from build123d import *

# Parameters (mm, degrees)
F1_DEPTH = 10
F3_DEPTH = 15
F4_R     = 0.99999


# Not quite as in the source:
# - a fillet or chamfer is up to 0.001 mm smaller than in the source, because OpenCascade refuses the exact size


with BuildPart() as f1:
    # F0 (on Top) → F1 (new body)
    with BuildSketch(Plane.XY):
        with BuildLine():
            ThreePointArc((-6.7175144213, -6.7175144213), (0, 9.5), (6.7175144213, -6.7175144213))
            Line((6.7175144213, -6.7175144213), (8.1317279836, -8.1317279836))
            ThreePointArc((8.1317279836, -8.1317279836), (11.4919258811, 0.430859077), (7.5, 8.7177978871))
            Line((7.5, 8.7177978871), (7.5, 9.5))
            Line((7.5, 9.5), (7.5, 14.5))
            Line((7.5, 14.5), (-7.5, 14.5))
            Line((-7.5, 14.5), (-7.5, 9.5))
            Line((-7.5, 9.5), (-7.5, 8.7177978871))
            ThreePointArc((-7.5, 8.7177978871), (-11.4919258811, 0.430859077), (-8.1317279836, -8.1317279836))
            Line((-8.1317279836, -8.1317279836), (-6.7175144213, -6.7175144213))
        make_face()
    extrude(amount=F1_DEPTH)

    # F2 (on face) → F3 (join, through all)
    with BuildSketch(Plane.YZ.offset(7.5)):
        with BuildLine():
            ThreePointArc((14.5, 5), (15.0465956117, 7.7117470016), (16.6010205144, 10))
            Line((16.6010205144, 10), (14.5, 10))
            Line((14.5, 10), (14.5, 5))
        make_face()
        with BuildLine():
            Line((14.5, 0), (16.6010205144, 0))
            ThreePointArc((16.6010205144, 0), (15.0465956117, 2.2882529984), (14.5, 5))
            Line((14.5, 5), (14.5, 0))
        make_face()
    extrude(amount=-F3_DEPTH)

    # F4 (radius 1 in the source; OpenCascade refuses exactly that, so slightly less here)
    f4_edges = [f1.edges().sort_by_distance(p)[0] for p in [
        (-6.717514, -6.717514, 5),
        (-8.131728, -8.131728, 5),
        (8.131728, -8.131728, 5),
        (6.717514, -6.717514, 5),
        (7.5, 8.717798, 5),
        (-7.5, 8.717798, 5),
    ]]
    fillet(f4_edges, radius=F4_R)


solid = f1.part
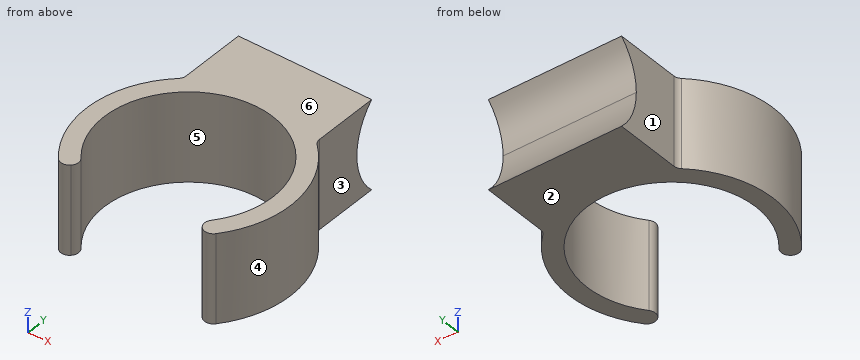
CAD build for the part. Positions are in the model's coordinates, mm. Face numbers are marked on the shaded views. A direction names the side the tool comes from. Round coordinates to 2 decimals unless told otherwise and drop trailing zeros. Write each loop counter-clockwise with the first axis right and the second up, starting at its lowest first coordinate (ties: lowest second). Pieces come first, ordered by that corner, then holes.
(1) Probe line 1 along X through (y, z) = (-0.25, 9.5); line 2 along X through (y, z) = (-2, 4.5); line 3 along Y through (x, z) = (-4, 2). List the from-to ranges inside material, lowest first.
(2) Slice it at A-A, the plane y = 0. Write the cut outline in (x, z).
(3) Mould opens along Y. For the marked faces 4, 5 and 6 say: pulls with the +Y half, pulls with the -Y half, needs draft (parallel to the pull), parting line crosses it, or undercut.
(4) Drop flat-ended pins along their axis: P1, Ø6, axis at x = 1.5, z = 3.5, coming from the -Y side; P2, Ø2, axis at x = 1.5, z = 6.5, coming from the -Y side; P3, Ø3, axis at x = 3.5, z = 7, coming from the -Y side. Give the stop position or say it passes through.
(5) 3-axis set-ups, long thin cutter, end or side, ignore diameter. For the marked faces 1, 2 and 3: which of +Z, -Z, +X, -X, +Y, -Y reach the whole face in a straight line?
(6) Slice it at D-D, the plane y = 11.25. Write the cut outline in (x, z), and give its area (3 significant figures).
(7) Slice it at B-B, the plane x = 0. Write the cut outline in (y, z).
From the geometry:
1. line 1: x = -11.5 to -9.5, 9.5 to 11.5
1. line 2: x = -11.32 to -9.29, 9.29 to 11.32
1. line 3: y = 8.62 to 15.18
2. outline: (-11.5, 0) - (-9.5, 0) - (-9.5, 10) - (-11.5, 10) - close; (9.5, 0) - (11.5, 0) - (11.5, 10) - (9.5, 10) - close
3. face 4: parting line crosses it
3. face 5: undercut
3. face 6: needs draft
4. P1: stops at y = 8.37
4. P2: stops at y = 9.17
4. P3: stops at y = 8.08
5. face 1: +Z, -Z, -X, +Y
5. face 2: -Z, +X, -X, +Y, -Y
5. face 3: +Z, -Z, +X, +Y
6. outline: (-7.5, 0) - (7.5, 0) - (7.5, 10) - (-7.5, 10) - close
6. area: 150 mm2
7. outline: (9.5, 0) - (16.6, 0) arc R7 cw to (16.6, 10) - (9.5, 10) - close
